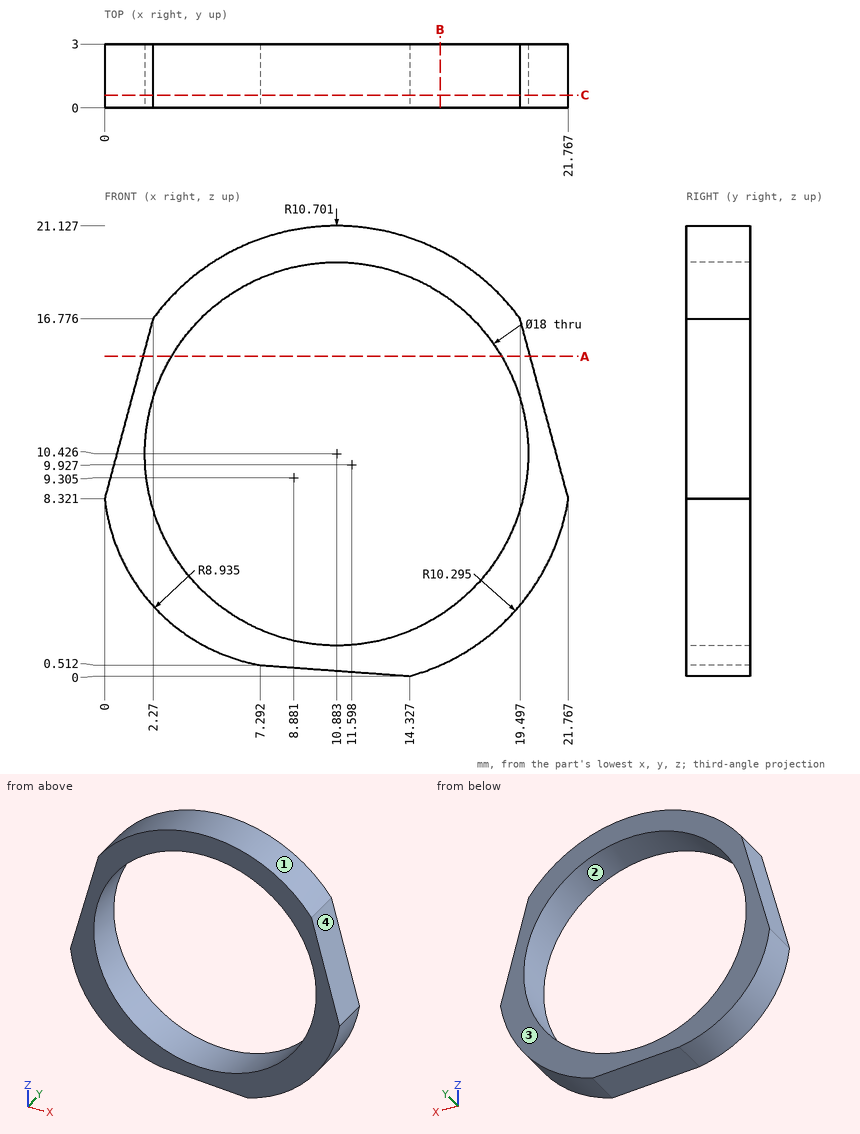
Job drawing, mm, ordinate dimensions from the low corner. One solid piece. Coordinates: 2 decimals unless noted, no trailing zeros. Order: outer loops, then holes, each group sorted by start corner. A loop starts at its lowest first (then second) coordinate and runs counter-clockwise, first axis right, second up. Notation, with made-up numbers: (76.5, 25.25) -> (121.5, 25.25) arc R24 ccw to (121.5, 42.25) -> close; hole circle Ø8 at (-12.75, 22.25). An arc over 180 degrees is marked (long way). Return JSON: item names as keys, results as strings. Group by question number.
Item 1: Flat gauge pins, fed straight in: P1, Ø1, axis at y = 2.5, z = 5.5, coming from the -X side; P2, Ø1, axis at y = 2, z = 13, coming from the +X side (1 decimal). Where does each tip first touch, or does it go through?
Item 2: Wall check: line 1 along X through (y, z) = (1.1, 15) (1 decimal); line 2 along X through (y, z) = (1.75, 8.5) (1 decimal); line 3 along Z through (x, y) = (12, 0.3) (1 decimal). Give the ranges that are in metal, low to high. Write a range as [from, to].
Item 3: Saw through at C-C on y = 0.6. Write the cut outline in (x, z) (1 decimal).
Item 4: Saw through at B-B on x = 15.75. Write the cut outline in (y, z) (1 decimal).
Item 5: Saw through at A-A on z = 15. Write the cut outline in (x, y) (1 decimal).
Item 6: Pull direction X, two halves, no side cores. Call the marked faces 1, 2, 3 and 4: pulls with the +X half, pulls with the -X half, needs draft (parallel to the pull), parting line crosses it, or undercut.
Values found:
{
 "1": {"P1": "stops at x = 0.58", "P2": "stops at x = 20.6"},
 "2": {"line 1": "x = [1.8, 3.1], [18.6, 20]", "line 2": "x = [0, 2.1], [19.7, 21.7]", "line 3": "z = [0.2, 1.5], [19.4, 21.1]"},
 "3": {"outline": "(0, 8.3) arc R8.9 ccw to (7.3, 0.5) -> (14.3, 0) arc R10.3 ccw to (21.8, 8.3) -> (19.5, 16.8) arc R10.7 ccw to (2.3, 16.8) -> close; hole circle Ø18 at (10.9, 10.4)"},
 "4": {"outline": "(0, 0.5) -> (3, 0.5) -> (3, 2.9) -> (0, 2.9) -> close; (0, 18) -> (3, 18) -> (3, 20) -> (0, 20) -> close"},
 "5": {"outline": "(1.8, 0) -> (3.1, 0) -> (3.1, 3) -> (1.8, 3) -> close; (18.6, 0) -> (20, 0) -> (20, 3) -> (18.6, 3) -> close"},
 "6": {"face 1": "parting line crosses it", "face 2": "undercut", "face 3": "needs draft", "face 4": "pulls with the +X half"}
}
